Can you work these out from the model? Positions are in its coordinate system, mm. Coordinates: 2 decimals unless noted, no trailing zeros. Write each loop counter-clockwise with the first axis right and the second up, starting at its lowest first coordinate (ties: lowest second). Pieces come first, ordered by that corner, then holes. Notation, with made-up numbers: (-25.5, 39.25) -> (-4.5, 39.25) arc R13 ccw to (-4.5, 54.25) -> close; hole circle Ø1 at (-12, 73.5). An arc over 180 degrees is marked (long way). Use one line per item in the form item = value.
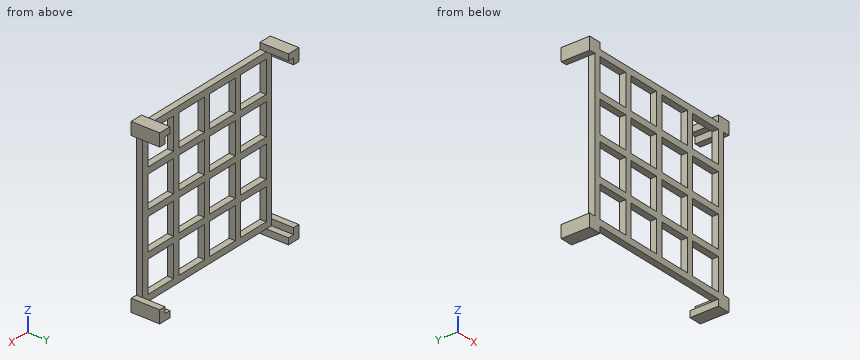
```python
from build123d import *

# Parameters (mm, degrees)
BOSS_EXTRUDE16_START   = 2
BOSS_EXTRUDE16_DEPTH   = 9
BOSS_EXTRUDE16_2_DEPTH = 9
BOSS_EXTRUDE16_3_DEPTH = 9
BOSS_EXTRUDE16_4_DEPTH = 9
BOSS_EXTRUDE17_START   = 2
SKETCH1_28_W           = 10
SKETCH1_28_H           = 10
BOSS_EXTRUDE17_DEPTH   = 2


with BuildPart() as part:
    # Sketch1 → Boss-Extrude16 (new body)
    with BuildSketch(Plane(origin=(0, 0, 0), x_dir=(1, 0, 0), z_dir=(0, 1, 0)).offset(BOSS_EXTRUDE16_START)):
        Polygon((4, 33), (4, 31), (6, 31), (6, 29), (8, 29), (8, 33), align=None)
    extrude(amount=BOSS_EXTRUDE16_DEPTH)



with BuildPart() as body_2:
    # Sketch1 → Boss-Extrude16 2 (new body)
    with BuildSketch(Plane(origin=(0, 0, 0), x_dir=(1, 0, 0), z_dir=(0, 1, 0)).offset(BOSS_EXTRUDE16_START)):
        Polygon((8, -17), (6, -17), (6, -19), (4, -19), (4, -21), (8, -21), align=None)
    extrude(amount=BOSS_EXTRUDE16_2_DEPTH)


with BuildPart() as body_3:
    # Sketch1 → Boss-Extrude16 3 (new body)
    with BuildSketch(Plane(origin=(0, 0, 0), x_dir=(1, 0, 0), z_dir=(0, 1, 0)).offset(BOSS_EXTRUDE16_START)):
        Polygon((-44, -19), (-44, -17), (-46, -17), (-46, -21), (-42, -21), (-42, -19), align=None)
    extrude(amount=BOSS_EXTRUDE16_3_DEPTH)


with BuildPart() as body_4:
    # Sketch1 → Boss-Extrude16 4 (new body)
    with BuildSketch(Plane(origin=(0, 0, 0), x_dir=(1, 0, 0), z_dir=(0, 1, 0)).offset(BOSS_EXTRUDE16_START)):
        Polygon((-44, 31), (-42, 31), (-42, 33), (-46, 33), (-46, 29), (-44, 29), align=None)
    extrude(amount=BOSS_EXTRUDE16_4_DEPTH)


with BuildPart() as part_1:
    add(part.part)

    add(body_2.part)  # Boss-Extrude17 merges body 2

    add(body_3.part)  # Boss-Extrude17 merges body 3

    add(body_4.part)  # Boss-Extrude17 merges body 4
    # Sketch1<28> → Boss-Extrude17 (add)
    with BuildSketch(Plane(origin=(0, 0, 0), x_dir=(1, 0, 0), z_dir=(0, 1, 0)).offset(BOSS_EXTRUDE17_START)):
        Polygon((4, 31), (-42, 31), (-44, 31), (-44, 29), (-44, -17), (-44, -19), (-42, -19), (4, -19), (6, -19), (6, -17), (6, 29), (6, 31), align=None)
        with Locations((-37, -12)):
            Rectangle(SKETCH1_28_W, SKETCH1_28_H, mode=Mode.SUBTRACT)
        with Locations((-25, -12)):
            Rectangle(SKETCH1_28_W, SKETCH1_28_H, mode=Mode.SUBTRACT)
        with Locations((-37, 0)):
            Rectangle(SKETCH1_28_W, SKETCH1_28_H, mode=Mode.SUBTRACT)
        with Locations((-25, 0)):
            Rectangle(SKETCH1_28_W, SKETCH1_28_H, mode=Mode.SUBTRACT)
        with Locations((-13, -12)):
            Rectangle(SKETCH1_28_W, SKETCH1_28_H, mode=Mode.SUBTRACT)
        with Locations((-1, -12)):
            Rectangle(SKETCH1_28_W, SKETCH1_28_H, mode=Mode.SUBTRACT)
        with Locations((-13, 0)):
            Rectangle(SKETCH1_28_W, SKETCH1_28_H, mode=Mode.SUBTRACT)
        with Locations((-1, 0)):
            Rectangle(SKETCH1_28_W, SKETCH1_28_H, mode=Mode.SUBTRACT)
        with Locations((-37, 12)):
            Rectangle(SKETCH1_28_W, SKETCH1_28_H, mode=Mode.SUBTRACT)
        with Locations((-25, 12)):
            Rectangle(SKETCH1_28_W, SKETCH1_28_H, mode=Mode.SUBTRACT)
        with Locations((-37, 24)):
            Rectangle(SKETCH1_28_W, SKETCH1_28_H, mode=Mode.SUBTRACT)
        with Locations((-25, 24)):
            Rectangle(SKETCH1_28_W, SKETCH1_28_H, mode=Mode.SUBTRACT)
        with Locations((-13, 12)):
            Rectangle(SKETCH1_28_W, SKETCH1_28_H, mode=Mode.SUBTRACT)
        with Locations((-1, 12)):
            Rectangle(SKETCH1_28_W, SKETCH1_28_H, mode=Mode.SUBTRACT)
        with Locations((-13, 24)):
            Rectangle(SKETCH1_28_W, SKETCH1_28_H, mode=Mode.SUBTRACT)
        with Locations((-1, 24)):
            Rectangle(SKETCH1_28_W, SKETCH1_28_H, mode=Mode.SUBTRACT)
    extrude(amount=BOSS_EXTRUDE17_DEPTH)


solid = part_1.part
```
Q1. If I drill on line 1 (Z direction, x = -12.5, y = 3); line 2 (X direction, y = 3, z = -27); line 3 (Y direction, x = -10, z = 6.5), over which ranges is the centre line in solid material (lowest first)? Write a range as from..to.
Return value:
line_1 = -31..-29, -19..-17, -7..-5, 5..7, 17..19
line_2 = -44..-42, -32..-30, -20..-18, -8..-6, 4..6
line_3 = 2..4
Q2. Suppose I cut it at B-B (y = 8.25). Write out the boundary of the cut face in (x, z).
Return value:
outline = (-46, -33) -> (-42, -33) -> (-42, -31) -> (-44, -31) -> (-44, -29) -> (-46, -29) -> close; (-46, 17) -> (-44, 17) -> (-44, 19) -> (-42, 19) -> (-42, 21) -> (-46, 21) -> close; (4, -33) -> (8, -33) -> (8, -29) -> (6, -29) -> (6, -31) -> (4, -31) -> close; (4, 19) -> (6, 19) -> (6, 17) -> (8, 17) -> (8, 21) -> (4, 21) -> close
Q3. Suppose I cut it at C-C (x = -34.5). Write out the boundary of the cut face in (y, z), then the cut area to 3 significant figures.
Return value:
outline = (2, -31) -> (4, -31) -> (4, -29) -> (2, -29) -> close; (2, -19) -> (4, -19) -> (4, -17) -> (2, -17) -> close; (2, -7) -> (4, -7) -> (4, -5) -> (2, -5) -> close; (2, 5) -> (4, 5) -> (4, 7) -> (2, 7) -> close; (2, 17) -> (4, 17) -> (4, 19) -> (2, 19) -> close
area = 20.0 mm2
Q4. Suppose I cut it at D-D (x = 5). Write out the boundary of the cut face in (y, z), then the cut area to 3 significant figures.
Return value:
outline = (2, -33) -> (11, -33) -> (11, -31) -> (4, -31) -> (4, 19) -> (11, 19) -> (11, 21) -> (2, 21) -> close
area = 136 mm2
Q5. Suppose I cut it at A-A (z = -26). Write out the boundary of the cut face in (x, y), then the cut area to 3 significant figures.
Return value:
outline = (-44, 2) -> (-42, 2) -> (-42, 4) -> (-44, 4) -> close; (-32, 2) -> (-30, 2) -> (-30, 4) -> (-32, 4) -> close; (-20, 2) -> (-18, 2) -> (-18, 4) -> (-20, 4) -> close; (-8, 2) -> (-6, 2) -> (-6, 4) -> (-8, 4) -> close; (4, 2) -> (6, 2) -> (6, 4) -> (4, 4) -> close
area = 20.0 mm2
Q6. Will these pins go through, and if not, where does the flat tip stop? pin 1 (6 mm diameter, centred on x = -36.5, z = -21, fed in from +Y); pin 2 (2 mm diameter, centred on y = 3, z = -17, fed in from -X); pin 3 (1 mm diameter, centred on x = -2.5, y = 4, fed in from -Z).
Return value:
pin_1 = 4
pin_2 = -44
pin_3 = -31
